For this review, take the finished solid that the model builds, in its own axes (mm). Face numbers are marked on the shaded views. A direction names the side the tool comes from. Give positions to 0.01 mm unless a question says otherwise; leave off trailing zeros. Write each loop counter-clockwise with the first axis right and the second up, starting at its lowest first coordinate (ties: lowest second). Pieces come first, ordered by that corner, then holes. Notation, with made-up numbers: M 74.5,86 L 111.5,86 A31 ccw 111.5,122 Z; hole C 8.25,-40 d5. An arc over 180 degrees is marked long. Use one line per item in the form item = value. Start each with the question number.
Q1. Tool access review of the marked faces 4, 5 and 6: name each direction out of +Z, -Z, +X, -X, +Y, -Y from which nothing blocks a thin tool from reaching the whole face with its end or side.
Q2. For probe 1 along X at (y, z) = (0, -15.25); probe 2 along Y at (x, z) = (0, -12) (3 decimals); probe 3 along Z at (x, y) = (69.5, -11), list the stretches that pass through material, from the lowest coordinate up. Write a range as [from, to].
Q3. Consider section A-A on z = -16.5. Write out the cut boundary in (x, y) (3 decimals), and give its area (3 significant figures).
Q4. Clearance check with flat-ended pins moving along their axes: pin 1 Ø1.5 at (y, z) = (58.5, -32) entering from +X; pin 2 Ø5 at (y, z) = (-38.5, -4.5) entering from +X; pin 3 Ø2.5 at (x, y) = (7.5, -64.5) entering from -Z; pin 4 Ø20.5 at (y, z) = (2, -15.5) entering from +X. State where each tip first meets the part, or that it passes through.
Q5. Consider section D-D on x = -59. Write out the cut boundary in (y, z).
Q6. Consider section B-B on x = 10. Write out the cut boundary in (y, z), and give its area (3 significant figures).
Q7. Consider section C-C on y = 25. Write out the cut boundary in (x, z), and give its area (3 significant figures).
Q8. Mouldability with a two-part tool opening along Y and no side actions: class the marked faces 1, 2 and 3 as released by +Y, released by -Y, zero draft, split by the parting line, or undercut.
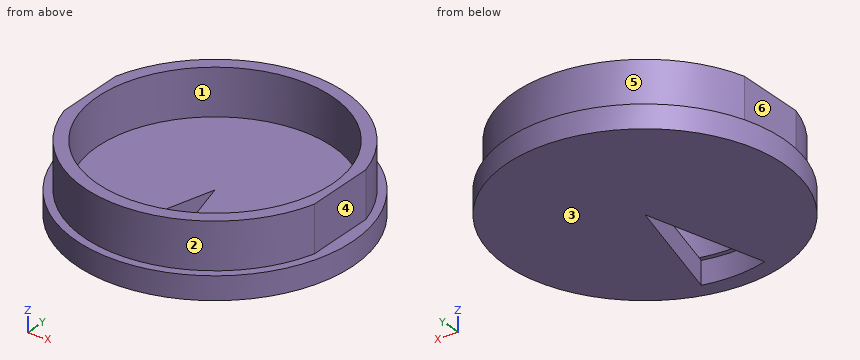
```python
from build123d import *

# Parameters (mm, degrees)
F0_R      = 76.2
F1_DEPTH  = 88.9
F2_R      = 76.2
F2_R_2    = 71.755
F3_DEPTH  = 25.4
F4_R      = 64.77
F5_DEPTH  = 25.4
F11_DEPTH = 63.501
F13_DEPTH = 25.4
F14_R     = 106.3100734062
F15_DEPTH = 50.8


with BuildPart() as f1:
    # F0 (on Top) → F1 (new body)
    with BuildSketch(Plane.XY):
        Circle(F0_R)
    extrude(amount=-F1_DEPTH)

    # F2 (on face) → F3 (cut)
    with BuildSketch(Plane.XY):
        Circle(F2_R)
        Circle(F2_R_2, mode=Mode.SUBTRACT)
    extrude(amount=-F3_DEPTH, mode=Mode.SUBTRACT)

    # F4 (on face) → F5 (cut)
    with BuildSketch(Plane.XY):
        Circle(F4_R)
    extrude(amount=-F5_DEPTH, mode=Mode.SUBTRACT)

    # F7 (on offset) → F11 (cut, through all)
    with BuildSketch(Plane.XY.offset(-25.4)):
        with BuildLine():
            Line((17.5278273627, -64.9877786045), (0, 0))
            Line((0, 0), (-17.5278273627, -64.9877786045))
            ThreePointArc((-17.5278273627, -64.9877786045), (0, -67.31), (17.5278273627, -64.9877786045))
        make_face()
    extrude(amount=-F11_DEPTH, mode=Mode.SUBTRACT)

    # F12 (on face) → F13 (cut)
    with BuildSketch(Plane.XY):
        with BuildLine():
            Line((-69.180037041, 0), (-69.180037041, 19.05))
            ThreePointArc((-69.180037041, 19.05), (-71.755, 0), (-69.180037041, -19.05))
            Line((-69.180037041, -19.05), (-69.180037041, 0))
        make_face()
        with BuildLine():
            ThreePointArc((71.755, 0), (71.1083454416, 9.6116197157), (69.180037041, 19.05))
            Line((69.180037041, 19.05), (69.180037041, 0))
            Line((69.180037041, 0), (69.180037041, -19.05))
            ThreePointArc((69.180037041, -19.05), (71.1083454416, -9.6116197157), (71.755, 0))
        make_face()
    extrude(amount=-F13_DEPTH, mode=Mode.SUBTRACT)

    # F14 (on face) → F15 (cut)
    with BuildSketch(Plane(origin=(0, 0, -88.9), x_dir=(1, 0, 0), z_dir=(0, 0, -1))):
        Circle(F14_R)
    extrude(amount=-F15_DEPTH, mode=Mode.SUBTRACT)


solid = f1.part
```
Working result:
q1.face_4 = +Z, +X, +Y, -Y
q1.face_5 = +Z, +Y
q1.face_6 = +Z, -X, +Y, -Y
q2.probe_1 = [-69.18, -64.77], [64.77, 69.18]
q2.probe_2 = [-71.755, -64.77], [64.77, 71.755]
q2.probe_3 = [-38.1, -25.4]
q3.outline = M -69.18,-19.05 A71.755 ccw 69.18,-19.05 L 69.18,19.05 A71.755 ccw -69.18,19.05 Z; hole C 0,0 d129.54
q3.area = 2,860 mm²
q4.pin_1 = 49.71
q4.pin_2 = 62.07
q4.pin_3 = -25.4
q4.pin_4 = 76.2
q5.outline = M -48.22,-38.1 L 48.22,-38.1 L 48.22,-25.4 L 40.84,-25.4 L 40.84,0 L 26.72,0 L 26.72,-25.4 L -26.72,-25.4 L -26.72,0 L -40.84,0 L -40.84,-25.4 L -48.22,-25.4 Z
q6.outline = M -75.54,-38.1 L -66.56,-38.1 L -66.56,-25.4 L -63.99,-25.4 L -63.99,0 L -71.05,0 L -71.05,-25.4 L -75.54,-25.4 Z; M -37.08,-38.1 L 75.54,-38.1 L 75.54,-25.4 L 71.05,-25.4 L 71.05,0 L 63.99,0 L 63.99,-25.4 L -37.08,-25.4 Z
q6.area = 1,900 mm²
q7.outline = M -71.98,-38.1 L 71.98,-38.1 L 71.98,-25.4 L 67.26,-25.4 L 67.26,0 L 59.75,0 L 59.75,-25.4 L -59.75,-25.4 L -59.75,0 L -67.26,0 L -67.26,-25.4 L -71.98,-25.4 Z
q7.area = 2,210 mm²
q8.face_1 = undercut
q8.face_2 = released by -Y
q8.face_3 = zero draft
